The listing builds one solid part. Answer for the finished solid, in the listing's coordinates (mm). A direction names the side the tool comes from. Give positions to 0.01 mm unless a question says otherwise; leave off trailing zeros. Loops run counter-clockwise (first coordinate to the right, second up) from the corner with the lowest first, then second, coordinate; pieces in that order, holes last. Notation, with made-up numbers: (18.5, -1) - (43.5, -1) arc R27 ccw to (43.5, 21) - close; hole circle Ø3 at (33, -15). An arc over 180 degrees is marked (long way). Write each question's results on one line, items separated by ' | '.
Autodesk Inventor part; units mm, degrees
ref_plane "YZ Plane" through (0, 0, 0) normal (1, 0, 0) x (0, 1, 0)
ref_plane "XZ Plane" through (0, 0, 0) normal (0, 1, 0) x (-1, 0, 0)
ref_plane "XY Plane" through (0, 0, 0) normal (0, 0, 1) x (1, 0, 0)
sketch "スケッチ1" plane through (0, 0, 0) normal (0, 1, 0) x (-1, 0, 0)
  line L0 (0, 0) -> (37, 0)
  line L1 (37, 0) -> (37, -22)
  line L2 (37, -22) -> (0, -22)
  line L3 (0, -22) -> (0, 0)
  line L4 (37, 0) -> (37, -3.6217)
  line L5 (37, 0) -> (32, 0)
  line L6 (32, 0) -> (32, -5)
  line L7 (32, -5) -> (37, -5)
  line L8 (37, -5) -> (37, 0)
  circle A0 centre (32, -5) radius 5
  line L9 (37, -22) -> (32, -22)
  line L10 (32, -22) -> (32, -17)
  line L11 (32, -17) -> (37, -17)
  line L12 (37, -17) -> (37, -22)
  circle A1 centre (32, -17) radius 5
  dimension "d1" = 22
  dimension "d2" = 37
  dimension "d6" = 5
  dimension "d7" = 5
extrude "押し出し1" add sketch "スケッチ1" along normal blind 19 contours L0 A0 L1 A1 L2 L3 | A0 L7 L6 | L6 L7 A0 | A1 L11 L10 | L10 L11 A1
sketch "スケッチ2" plane through (0, 19, 0) normal (0, 1, 0) x (1, 0, 0)
  line L0 (0, 0) -> (0, 22)
  line L1 (0, 0) -> (0, 22)
  line L2 (0, 11) -> (-37, 11)
  line L3 (-37, 17) -> (-37, 5)
  line L4 (-37, 11) -> (-26, 11)
  circle A0 centre (-26, 11) radius 2.75
  line L5 (-28, 9.1125) -> (-24, 9.1125)
  line L6 (-28, 12.8875) -> (-24, 12.8875)
  dimension "d10" = 11
  dimension "d11" = 5.5
  dimension "d12" = 4
extrude "押し出し2" add sketch "スケッチ2" along normal blind 8 contours A0 L5 L2 | L2 A0 L6
sketch "スケッチ3" plane through (0, 0, 0) normal (0, -1, 0) x (1, 0, 0)
  arc A0 (-24, -12.8875) -> (-24, -9.1125) centre (-26, -11) ccw
  line L0 (-28, -12.8875) -> (-24, -12.8875)
  arc A1 (-28, -9.1125) -> (-28, -12.8875) centre (-26, -11) ccw
  line L1 (-24, -9.1125) -> (-28, -9.1125)
  point P0 (0, 0)
extrude "押し出し3" add sketch "スケッチ3" along normal blind 8
sketch "スケッチ4" plane through (0, 19, 0) normal (0, 1, 0) x (1, 0, 0)
  line L0 (0, 0) -> (0, 22)
  line L1 (0, 11) -> (-15, 11)
  circle A0 centre (-15, 11) radius 2
  dimension "d17" = 15
  dimension "d18" = 4
extrude "押し出し4" add sketch "スケッチ4" along normal blind 2
sketch "スケッチ5" plane through (0, 0, 0) normal (1, 0, 0) x (0, 0, -1)
  line L0 (22, 0) -> (22, 19)
  line L1 (0, 0) -> (22, 0)
  line L2 (22, 0) -> (22, 18)
  line L3 (22, 18) -> (0, 18)
  line L4 (0, 18) -> (0, 0)
  line L5 (0, 0) -> (0, 19)
  line L6 (0, 9) -> (22, 9)
  line L7 (11, 0) -> (11, 18)
  line L8 (4, 9) -> (4, 0)
  ellipse E0 centre (4, 9) end of major axis (0, 9) minor radius 9
  ellipse E1 centre (18, 9) end of major axis (22, 9) minor radius 9
  point P0 (4, 18)
  point P1 (18, 0)
  point P2 (18, 18)
  dimension "d21" = 18
extrude "押し出し5" add sketch "スケッチ5" along normal blind 28 contours E1 L6 | L6 E1 | L1 L7 L6 E1 | L6 L7 L3 E1 | L1 E0 L6 L7 | L6 E0 L3 L7 | E0 L6 L8 | L8 L6 E0 | L6 E0
sketch "スケッチ6" plane through (0, 19, 0) normal (0, 1, 0) x (1, 0, 0)
  arc A0 (-32, 22) -> (-37, 17) centre (-32, 17) ccw
  line L0 (0, 0) -> (0, 22)
  line L1 (-32, 22) -> (0, 22)
  line L2 (0, 22) -> (-2.4665, 22)
  line L3 (0, 0) -> (-5.5, 0)
  line L4 (-32, 0) -> (0, 0)
  line L5 (-5.5, 0) -> (-5.5, 2.5)
  circle A1 centre (-5.5, 2.5) radius 1.5
  line L6 (0, 11) -> (-37, 11)
  line L7 (-37, 17) -> (-37, 5)
  circle A2 centre (-5.5, 19.5) radius 1.5
  dimension "d25" = 5.5
  dimension "d26" = 2.5
  dimension "d27" = 3
extrude "押し出し6" cut sketch "スケッチ6" against normal blind 22 contours A1 | A2
properties part number "黄モーター"
Item 1: For faces 4 (the face through (-15, 21, -11)), 5 (the face through (-15, 20, -9)), 6 (the face through (-26, -4, -9.112)), 7 (the face through (0, 18.8, -11.1)), determine the directions among +Z, -Z, +X, -X, +Y, -Y from which every point of the face is accessible in a straight line to the end or side of a thin tool.
Values found:
face 4: +Z, -Z, +X, +Y | face 5: +Y | face 6: +Z, +X, -X, -Y | face 7: +X, +Y
Item 2: A cutting plane is placed at B-B, the plane x = -15. Determine the outline of the cut face in (y, z), plus the area to 3 significant figures.
Values found:
outline: (0, -22) - (19, -22) - (19, -13) - (21, -13) - (21, -9) - (19, -9) - (19, 0) - (0, 0) - close | area: 426 mm²
Item 3: A cutting plane is placed at A-A, the plane x = -5.5. Determine the outline of the cut face in (y, z), plus the area to 3 significant figures.
Values found:
outline: (0, -22) - (19, -22) - (19, -21) - (0, -21) - close; (0, -18) - (19, -18) - (19, -4) - (0, -4) - close; (0, -1) - (19, -1) - (19, 0) - (0, 0) - close | area: 304 mm²
Item 4: Flat-ended cylindrical pins translate along their axes: P1, Ø10, axis at x = 21.5, z = -11.5, coming from the +Y side; P2, Ø1.2, axis at x = -26, y = -4, coming from the -Z side; P3, Ø1.2, axis at x = -14.5, z = -12, coming from the +Y side; P4, Ø2.5, axis at x = -5.5, z = -2.5, coming from the +Y side. Find the tip coordinate at first contact, or state that the pin passes through.
Values found:
P1: stops at y = 18 | P2: stops at z = -12.89 | P3: stops at y = 21 | P4: passes through
Item 5: A cutting plane is placed at D-D, the plane y = 1. Count the separate pieces of the cut face and the enclosed holes in it, plus the area to 3 significant figures.
Values found:
separate pieces: 1 | enclosed holes: 2 | area: 1,280 mm²
Item 6: Find the intervals of material crossed by line 1 along Z through (x, y) = (-5.5, 15.25); line 2 along Z through (x, y) = (-5, 10); line 3 along Y through (x, z) = (15, -9.5), in increasing order. Write a range as [from, to].
Values found:
line 1: z = [-22, -21], [-18, -4], [-1, 0] | line 2: z = [-22, -20.91], [-18.09, -3.91], [-1.09, 0] | line 3: y = [0, 18]
Item 7: For a pull along X with two mould halves and no side action, classify faces 1 (the face through (-6.61, 9.63, -20.51)), 2 (the face through (0, 2, -1)), 3 (the face through (-28.75, -3.94, -11.03)) as released by +X, released by -X, zero draft, split by the parting line, or undercut.
Values found:
face 1: undercut | face 2: released by +X | face 3: released by -X
Item 8: A cutting plane is placed at C-C, the plane z = -11. Determine the outline of the cut face in (x, y).
Values found:
outline: (-37, 0) - (-28.75, 0) - (-28.75, -8) - (-23.25, -8) - (-23.25, 0) - (28, 0) - (28, 18) - (0, 18) - (0, 19) - (-13, 19) - (-13, 21) - (-17, 21) - (-17, 19) - (-23.25, 19) - (-23.25, 27) - (-28.75, 27) - (-28.75, 19) - (-37, 19) - close
